```python
from build123d import *

# Parameters (mm, degrees)
SKETCH1_R               = 60
BOSS_EXTRUDE1_DEPTH     = 25.1
SKETCH3_R               = 47.5
CUT_EXTRUDE2_DEPTH      = 14
CUT_EXTRUDE5_DEPTH      = 89.487343728
CUT_EXTRUDE5_DEPTH_BACK = 89.487343728
SKETCH2_R               = 2.494998654
SKETCH2_R_2             = 2.5
SKETCH2_R_3             = 2.444443829
SKETCH6_R               = 3
CUT_EXTRUDE6_DEPTH      = 6
CUT_EXTRUDE7_DEPTH      = 87
CUT_EXTRUDE7_DEPTH_BACK = 87
SKETCH8_R               = 2.5
CUT_EXTRUDE8_DEPTH      = 81
CUT_EXTRUDE9_DEPTH      = 3


with BuildPart() as part:
    # Sketch1 → Boss-Extrude1 (new body)
    with BuildSketch(Plane.XY):
        Circle(SKETCH1_R)
    extrude(amount=BOSS_EXTRUDE1_DEPTH)

    # Sketch3 → Cut-Extrude2 (cut)
    with BuildSketch(Plane.XY.offset(25.1)):
        Circle(SKETCH3_R)
    extrude(amount=-CUT_EXTRUDE2_DEPTH, mode=Mode.SUBTRACT)

    # Sketch2 → Cut-Extrude5 (cut, two sides: drawn at the far end of the back side and taken through both)
    with BuildSketch(Plane.XY.offset(25.1).offset(-CUT_EXTRUDE5_DEPTH_BACK)):
        with Locations((-16.664697145, -50.733104448)):
            Circle(SKETCH2_R)
        with Locations((-50.733105114, 16.664696544)):
            Circle(SKETCH2_R_2)
        with Locations((16.664695878, 50.733104512)):
            Circle(SKETCH2_R_3)
        with Locations((50.733103846, -16.66469648)):
            Circle(SKETCH2_R_2)
    extrude(amount=CUT_EXTRUDE5_DEPTH + CUT_EXTRUDE5_DEPTH_BACK, mode=Mode.SUBTRACT)

    # Sketch6 → Cut-Extrude6 (cut)
    with BuildSketch(Plane(origin=(0, 0, 0), x_dir=(-1, 0, 0), z_dir=(0, 0, -1))):
        with Locations((11.973502988, 47.212610548)):
            Circle(SKETCH6_R)
        with Locations((27.381285989, 40.029281029)):
            Circle(SKETCH6_R)
        with Locations((-19.717656658, -20.762902692)):
            Circle(SKETCH6_R)
        with Locations((-4.309873657, -27.946232212)):
            Circle(SKETCH6_R)
    extrude(amount=-CUT_EXTRUDE6_DEPTH, mode=Mode.SUBTRACT)

    # Sketch7 → Cut-Extrude7 (cut, two sides: drawn at the far end of the back side and taken through both)
    with BuildSketch(Plane.XY.offset(11.1).offset(-CUT_EXTRUDE7_DEPTH_BACK)):
        Polygon((-32.722381774, 32.714358343), (-3.845549598, -27.273283804), (24.859322702, -13.455341469), (-3.0425496, 47.001626555), align=None)
    extrude(amount=CUT_EXTRUDE7_DEPTH + CUT_EXTRUDE7_DEPTH_BACK, mode=Mode.SUBTRACT)

    # Sketch8 → Cut-Extrude8 (cut)
    with BuildSketch(Plane(origin=(0, 0, 0), x_dir=(-1, 0, 0), z_dir=(0, 0, -1))):
        with Locations((-39.427412605, -12.951028347)):
            Circle(SKETCH8_R)
        with Locations((-12.951028347, 39.427412605)):
            Circle(SKETCH8_R)
        with Locations((39.427412605, 12.951028347)):
            Circle(SKETCH8_R)
        with Locations((12.951028347, -39.427412605)):
            Circle(SKETCH8_R)
    extrude(amount=-CUT_EXTRUDE8_DEPTH, mode=Mode.SUBTRACT)

    # Sketch9 → Cut-Extrude9 (cut)
    with BuildSketch(Plane(origin=(0, 0, 0), x_dir=(-1, 0, 0), z_dir=(0, 0, -1))):
        Polygon((-8.880375106, -21.147282201), (-11.884100541, -27.387108141), (-14.440828659, -26.156351169), (-11.437103225, -19.916525229), align=None)
        Polygon((19.284340571, 39.183158361), (22.354381036, 45.560744644), (19.657241196, 46.859092966), (16.587200731, 40.481506683), align=None)
    extrude(amount=-CUT_EXTRUDE9_DEPTH, mode=Mode.SUBTRACT)


solid = part.part
```
CAD build for the part. Positions are in the model's coordinates, mm. A direction names the side the tool comes from. Round coordinates to 2 decimals unless told otherwise and drop trailing zeros. Order: outer loops, then holes, each group sorted by start corner. A loop starts at its lowest first (then second) coordinate and runs counter-clockwise, first axis right, second up.
Q1. Slice it at B-B (z = 23.5). Write the cut outline in (x, y) (3 decimals), and give its area (3 significant figures).
Q2. Slice it at D-D (y = 31). Write the cut outline in (x, z), and give its area (3 significant figures).
Q3. Slice it at C-C (z = 8). State how many separate pieces and enclosed holes the cut face has, and give its area (3 significant figures).
Q4. Drop flat-ended pins along their axis: pin 1 (3.5 mm diameter, centred on x = 4.31, y = -27.95, fed in from -Z); pin 2 (10 mm diameter, centred on x = -12, z = 18, fed in from -Y); pin 3 (1 mm diameter, centred on x = -32.5, z = 22, fed in from -Y). Give the stop position or say it passes through.
Q5. Two-plate mould, pull along X, no slides. Class faces 4 (the cylindrical face through (16.946, -21.912, 2.958)), 5 (the cylindrical face through (-11.323, 44.284, 2.958)), 6 (the flat face through (-5, -49, 25.1)), 7 (the cylindrical face through (-59.94, 2.64, 12.37)): pulls with the +X half, pulls with the -X half, needs draft (parallel to the pull), parting line crosses it, or undercut.
Q6. Wall check: L1, parallel to X at y = -25.5, z = 5.5; L2, parallel to X at y = -1, z = 23.75; L3, parallel to X at y = 18.5, z = 16.25. Give the ranges that are in metal, low to high.
Q7. Slice it at A-A (y = 0). Write the cut outline in (x, z), and give its area (3 significant figures).
Q8. Which spindle directions (+Z, -Z, +X, -X, +Y, -Y) get a long thin tool onto all of the face, cutting with end or side? Do faces 1 (the flat face through (11.104, 16.35, 5.472)), 2 (the cylindrical face through (4.96, -30.875, 2.958)), 3 (the flat face through (-14, -12, 0)). Say none if no direction does.
Results below:
1. outline: circle Ø120 at (0, 0); hole circle Ø5 at (-50.733, 16.665); hole circle Ø95 at (0, 0); hole circle Ø4.99 at (-16.665, -50.733); hole circle Ø4.889 at (16.665, 50.733); hole circle Ø5 at (50.733, -16.665)
1. area: 4,140 mm2
2. outline: (-51.37, 0) - (-31.9, 0) - (-31.9, 11.1) - (-35.99, 11.1) - (-35.99, 25.1) - (-51.37, 25.1) - close; (4.34, 0) - (51.37, 0) - (51.37, 25.1) - (35.99, 25.1) - (35.99, 11.1) - (4.34, 11.1) - close
2. area: 1,170 mm2
3. separate pieces: 1
3. enclosed holes: 9
3. area: 9,000 mm2
4. pin 1: stops at z = 6
4. pin 2: stops at y = -59.59
4. pin 3: stops at y = -50.75
5. face 4: undercut
5. face 5: undercut
5. face 6: needs draft
5. face 7: parting line crosses it
6. L1: x = -54.31 to -4.7, -0.16 to 2.57, 6.05 to 54.31
6. L2: x = -59.99 to -47.49, 47.49 to 59.99
6. L3: x = -57.08 to -52.43, -49.04 to -43.75, 43.75 to 57.08
7. outline: (-60, 0) - (-16.97, 0) - (-16.97, 11.1) - (-47.5, 11.1) - (-47.5, 25.1) - (-60, 25.1) - close; (18.65, 0) - (60, 0) - (60, 25.1) - (47.5, 25.1) - (47.5, 11.1) - (18.65, 11.1) - close
7. area: 1,290 mm2
8. face 1: +Z, -Z
8. face 2: -Z
8. face 3: -Z, +X, -X, +Y, -Y
